The figure shows three views and two pictorial views of one solid part (mm, origin at its lowest corner). Answer the questions. A direction names the side the tool comes from. Round coordinates to 2 decimals unless told otherwise and drop trailing zeros. Loops run counter-clockwise (first coordinate to the right, second up) from the corner with the lowest first, then second, coordinate; pieces in that order, holes last. Notation, with made-up numbers: (-29.5, 19.25) -> (7.5, 19.25) arc R20 cw to (7.5, 42.25) -> close; hole circle Ø5 at (-14.75, -34). An arc over 180 degrees is marked (long way). Put each result on its own line as item: value.
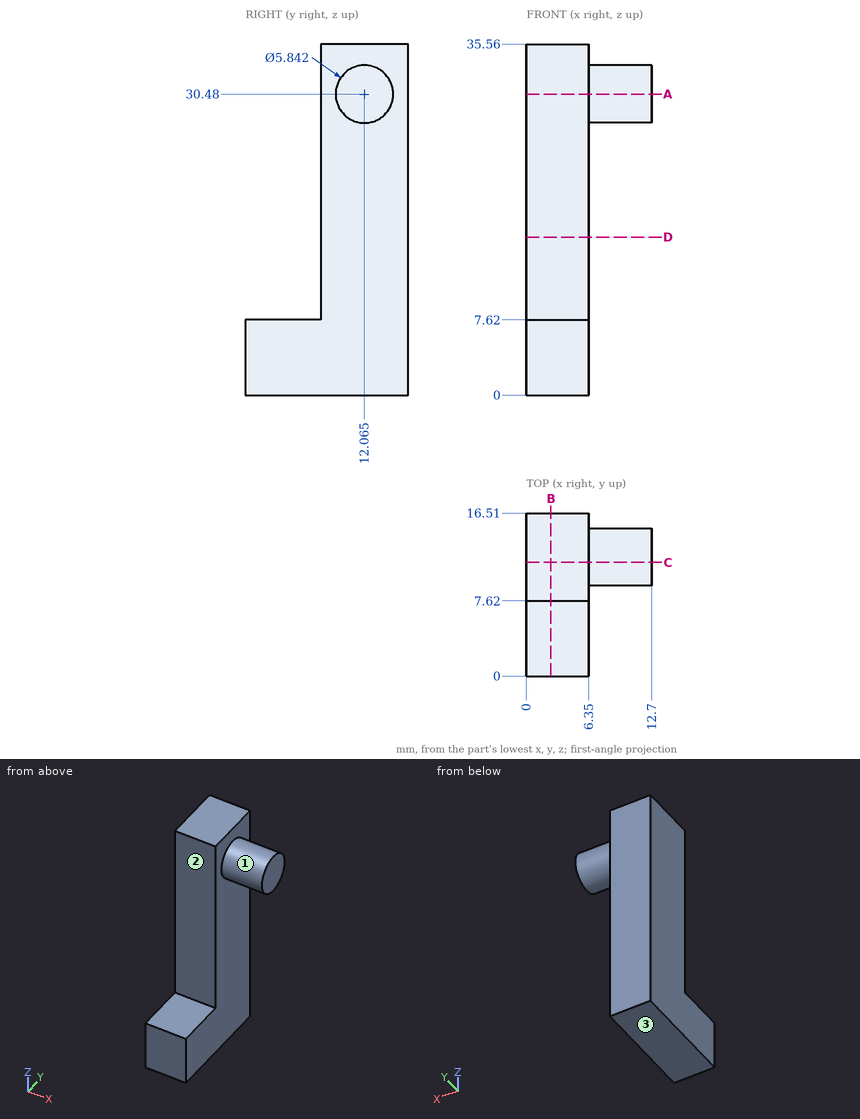
Item 1: The part is cut by section B-B (x = 2.5). Determine the outline of the cut face in (y, z).
Derived:
outline: (0, 0) -> (16.51, 0) -> (16.51, 35.56) -> (7.62, 35.56) -> (7.62, 7.62) -> (0, 7.62) -> close
Item 2: Which of the six approach directions +Z, -Z, +X, -X, +Y, -Y give full straight-line access (tool end or side, diameter ignored) to the marked faces 1, 2 and 3?
Derived:
face 1: +X
face 2: +Z, +X, -X, -Y
face 3: -Z, +X, -X, +Y, -Y
Item 3: The part is cut by section A-A (z = 30.48). Determine the outline of the cut face in (x, y), then the cut area to 3 significant figures.
Derived:
outline: (0, 7.62) -> (6.35, 7.62) -> (6.35, 9.14) -> (12.7, 9.14) -> (12.7, 14.99) -> (6.35, 14.99) -> (6.35, 16.51) -> (0, 16.51) -> close
area: 93.5 mm^2
Item 4: The part is cut by section D-D (z = 16). Determine the outline of the cut face in (x, y).
Derived:
outline: (0, 7.62) -> (6.35, 7.62) -> (6.35, 16.51) -> (0, 16.51) -> close
Item 5: The part is cut by section C-C (y = 11.5). Determine the outline of the cut face in (x, z).
Derived:
outline: (0, 0) -> (6.35, 0) -> (6.35, 27.61) -> (12.7, 27.61) -> (12.7, 33.35) -> (6.35, 33.35) -> (6.35, 35.56) -> (0, 35.56) -> close
Item 6: Flat-ended cylindrical pins translate along their axes: pin 1 Ø1.5 at (x, y) = (1.5, 4) entering from -Z; pin 2 Ø6 at (x, z) = (10, 3.5) entering from +Y; pin 3 Ø4 at (y, z) = (13, 11) entering from +X; pin 4 Ø1.9 at (x, z) = (2, 22) entering from -Y. Find the tip coordinate at first contact, or state that the pin passes through.
Derived:
pin 1: stops at z = 0
pin 2: passes through
pin 3: stops at x = 6.35
pin 4: stops at y = 7.62
Item 7: Find the intervals of material crossed by line 1 along X through (y, z) = (13.5, 16); line 2 along Y through (x, z) = (2.75, 28); line 3 along Z through (x, y) = (7.5, 12), in increasing order.
Derived:
line 1: x = 0 to 6.35
line 2: y = 7.62 to 16.51
line 3: z = 27.56 to 33.4
